```python
from build123d import *

# Parameters (mm, degrees)
SKETCH_W        = 100
SKETCH_H        = 25
PAD_DEPTH       = 8.6
SKETCH001_W     = 111.182612
SKETCH001_H     = 13.535424
POCKET_DEPTH    = 1.6
SKETCH002_R     = 2.75
POCKET001_DEPTH = 8.601
POCKET002_DEPTH = 4.5
SKETCH004_R     = 1.6
POCKET003_DEPTH = 8.601
POCKET004_DEPTH = 3.5
CHAMFER_SIZE    = 1


with BuildPart() as part:
    # Sketch → Pad (new body)
    with BuildSketch(Plane.XY):
        with Locations((50, 12.5)):
            Rectangle(SKETCH_W, SKETCH_H)
    extrude(amount=PAD_DEPTH)

    # Sketch001 → Pocket (cut)
    with BuildSketch(Plane.XY.offset(8.6)):
        with Locations((49.408694, 3.232288)):
            Rectangle(SKETCH001_W, SKETCH001_H)
    extrude(amount=-POCKET_DEPTH, mode=Mode.SUBTRACT)

    # Sketch002 → Pocket001 (cut, through all)
    with BuildSketch(Plane.XY.offset(8.6)):
        with Locations((50, 15)):
            Circle(SKETCH002_R)
    extrude(amount=-POCKET001_DEPTH, mode=Mode.SUBTRACT)

    # Sketch003 → Pocket002 (cut)
    with BuildSketch(Plane(origin=(0, 0, 0), x_dir=(1, 0, 0), z_dir=(0, 0, -1))):
        with BuildLine():
            ThreePointArc((33.459446, -27.93431), (33.459446, -31.540554), (37.06569, -31.540554))
            Line((37.06569, -31.540554), (71.803122, 3.196878))
            ThreePointArc((71.803122, 3.196878), (71.803122, 6.803122), (68.196878, 6.803122))
            Line((33.459446, -27.93431), (68.196878, 6.803122))
        make_face()
    extrude(amount=-POCKET002_DEPTH, mode=Mode.SUBTRACT)

    # Sketch004 → Pocket003 (cut, through all)
    with BuildSketch(Plane.XY.offset(8.6)):
        with Locations((70, 11.886219)):
            Circle(SKETCH004_R)
    extrude(amount=-POCKET003_DEPTH, mode=Mode.SUBTRACT)

    # Sketch005 → Pocket004 (cut)
    with BuildSketch(Plane(origin=(0, 0, 0), x_dir=(1, 0, 0), z_dir=(0, 0, -1))):
        Polygon((72.524127, -13.906643), (73.011802, -10.710473), (70.487675, -8.690048), (67.475873, -9.865795), (66.988198, -13.061965), (69.512325, -15.08239), align=None)
    extrude(amount=-POCKET004_DEPTH, mode=Mode.SUBTRACT)

    # Chamfer
    chamfer_edges = [part.edges().sort_by_distance(p)[0] for p in [
        (30.696878, 0, 0),
        (0, 0, 3.5),
        (0, 12.5, 0),
        (18.196878, 25, 0),
        (84.303122, 0, 0),
        (100, 12.5, 0),
        (100, 0, 3.5),
        (100, 25, 4.3),
        (71.803122, 25, 0),
        (100, 17.5, 8.6),
        (0, 25, 4.3),
        (0, 17.5, 8.6),
        (50, 25, 8.6),
    ]]
    chamfer(chamfer_edges, length=CHAMFER_SIZE)


solid = part.part
```
Here's how the part is built. I have some questions about the finished solid (model axes, mm). A direction names the side the tool comes from. Coordinates: 2 decimals unless noted, no trailing zeros. Loops run counter-clockwise (first coordinate to the right, second up) from the corner with the lowest first, then second, coordinate; pieces in that order, holes last. Notation, with made-up numbers: M 6,81 L 14,81 A26 cw 14,113 Z; hole C 43,89 d11. An arc over 180 degrees is marked long. One line per item, written item: value.
1. Thinking about a two-plate mould opening in X: for faces 3 (the flat face through (49, 5, 7)), 4 (the flat face through (68.233, 14.058, 1.726)), 5 (the flat face through (0, 12, 4)), 6 (the cylindrical face through (71.526, 12.367, 6.086)), which applies, +X half, -X half, draft (parallel to the pull), parting line (faces both ways), or undercut?
Geometry says:
face 3: draft
face 4: undercut
face 5: -X half
face 6: undercut
2. Imagine slicing it at C-C (y = 6.75). List the corners of the cut face in (x, z) for me.
Geometry says:
outline: M 0,1 L 1,0 L 54.64,0 L 54.64,4.5 L 61.86,4.5 L 61.86,0 L 99,0 L 100,1 L 100,7 L 0,7 Z
3. Will these pins go through, and if not, where does the flat tip stop? pin 1 Ø0.5 at (x, z) = (29, 7.5) entering from -Y; pin 2 Ø8 at (x, y) = (64, 4.5) entering from +Z.
Geometry says:
pin 1: stops at y = 10
pin 2: stops at z = 7
4. On a 3-axis mill with a long thin cutter (end or side, diameter ignored), from which of +Z, -Z, +X, -X, +Y, -Y can I reach the whole of each face in a straight line? I mean faces 1 (the flat face through (71, 14.5, 1.7)), 2 (the flat face through (77, 13, 0)). Say none if no direction works.
Geometry says:
face 1: -Z
face 2: -Z, +X, -X, +Y, -Y
5. Imagine slicing it at B-B (x = 34). List the corners of the cut face in (y, z) for me.
Geometry says:
outline: M 0,1 L 1,0 L 24,0 L 25,1 L 25,7.6 L 24,8.6 L 10,8.6 L 10,7 L 0,7 Z
6. Please list where these lines run through material, in increasing order: probe 1 along X at (y, z) = (15, 5.5); probe 2 along Y at (x, z) = (70, 5.9); probe 3 along Y at (x, z) = (50, 6.75).
Geometry says:
probe 1: x = 0 to 47.25, 52.75 to 100
probe 2: y = 0 to 10.29, 13.49 to 25
probe 3: y = 0 to 12.25, 17.75 to 25
7. Imagine slicing it at A-A (x = 50). List the corners of the cut face in (y, z) for me.
Geometry says:
outline: M 0,1 L 1,0 L 11.39,0 L 11.39,4.5 L 12.25,4.5 L 12.25,8.6 L 10,8.6 L 10,7 L 0,7 Z; M 17.75,4.5 L 18.61,4.5 L 18.61,0 L 24,0 L 25,1 L 25,7.6 L 24,8.6 L 17.75,8.6 Z
